from build123d import *

# Parameters (mm, degrees)
F1_DEPTH = 85
F3_D     = 4.2
F3_DEPTH = 14.4
F3_TIP   = 1.2618073
F5_D     = 3.2


with BuildPart() as f1:
    # F0 (on Front) → F1 (new body)
    with BuildSketch(Plane.XZ):
        Polygon((0, 37), (0, 0), (13.5, 0), (13.5, 23), (71.5, 23), (71.5, 0), (85, 0), (85, 37), align=None)
    extrude(amount=F1_DEPTH)

    # F3
    with Locations(Plane.XY.offset(37)):
        with Locations((11.7691496318, -12.5), (72.5, -12.5), (72.5, -72.5), (12.5, -72.5)):
            Hole(F3_D / 2, depth=F3_DEPTH)
            with Locations((0, 0, -(F3_DEPTH + F3_TIP / 2))):  # 118° drill point
                Cone(0, F3_D / 2, F3_TIP, mode=Mode.SUBTRACT)

    # F5 (through all)
    with Locations(Plane.YZ.offset(85)):
        with Locations((-57.5, 19), (-27.5, 19)):
            Hole(F5_D / 2)


solid = f1.part
Design review of the part built by this model. Coordinates are the model's own, in mm. A direction names the side the tool comes from. Give positions to 0.01 mm unless a question says otherwise; leave off trailing zeros. Loops run counter-clockwise (first coordinate to the right, second up) from the corner with the lowest first, then second, coordinate; pieces in that order, holes last. Notation, with made-up numbers: (63, 70.5) - (83, 70.5) arc R14 cw to (83, 83.5) - close; hole circle Ø1 at (-28.5, 54.5). An arc over 180 degrees is marked (long way). Use CSV: the item, a comma, the result in double quotes. Start each with the question number.
1. Add section A-A (y = -57.5). State the section outline as (x, z) points.
2. Wall thickness on L1, parallel to X at y = -12.5, z = 31.75; L2, parallel to X at y = -38.5, z = 18; L3, parallel to Z at x = 37, y = -67: over which ranges is each line inside the solid? List them lowest first.
3. Add section D-D (y = -36). State the section outline as (x, z) points, plus the area to 3 significant figures.
4. Insertion check: P1, Ø2.5, axis at x = 11.77, y = -12.5, coming from the +Z side; P2, Ø1.5, axis at x = 23.5, y = -71.5, coming from the -Z side. Each pin has a flat end and moves straight along its axis. Give the tip position at first contact, or say it passes through.
5. Add section C-C (z = 3.5). State the section outline as (x, y) points.
6. Draft analysis for pull direction Y (two halves, no side actions). For faces 4 (the cylindrical face through (9.766, -11.869, 29.699)), 5 (the flat face through (42, 0, 27)), 6 (the flat face through (42, -42, 23)), state which applies: released by +Y, released by -Y, zero draft, split by the parting line, or undercut.
7. Machinability: for faces 1 (the flat face through (85, -42, 18)), 2 (the flat face through (13.5, -42, 11)), 3 (the cylindrical face through (74.6, -12.41, 29.7)), which of the approach directions +Z, -Z, +X, -X, +Y, -Y give a long, thin tool a straight path to every point of the face, cutting with its end or side? Answer none if there is none.
8. Add section B-B (z = 19). State the section outline as (x, y) points, plus the area to 3 significant figures.
Results found:
1,outline,"(0, 0) - (13.5, 0) - (13.5, 17.4) - (0, 17.4) - close; (0, 20.6) - (13.5, 20.6) - (13.5, 23) - (71.5, 23) - (71.5, 20.6) - (85, 20.6) - (85, 37) - (0, 37) - close; (71.5, 0) - (85, 0) - (85, 17.4) - (71.5, 17.4) - close"
2,L1,"x = 0 to 9.67, 13.87 to 70.4, 74.6 to 85"
2,L2,"x = 0 to 13.5, 71.5 to 85"
2,L3,"z = 23 to 37"
3,outline,"(0, 0) - (13.5, 0) - (13.5, 23) - (71.5, 23) - (71.5, 0) - (85, 0) - (85, 37) - (0, 37) - close"
3,area,"1,810 mm²"
4,P1,"stops at z = 22.09"
4,P2,"stops at z = 23"
5,outline,"(0, -85) - (13.5, -85) - (13.5, 0) - (0, 0) - close; (71.5, -85) - (85, -85) - (85, 0) - (71.5, 0) - close"
6,face 4,"undercut"
6,face 5,"released by +Y"
6,face 6,"zero draft"
7,face 1,"+Z, -Z, +X, +Y, -Y"
7,face 2,"-Z, +Y, -Y"
7,face 3,"+Z"
8,outline,"(0, -85) - (13.5, -85) - (13.5, -59.1) - (0, -59.1) - close; (0, -55.9) - (13.5, -55.9) - (13.5, -29.1) - (0, -29.1) - close; (0, -25.9) - (13.5, -25.9) - (13.5, 0) - (0, 0) - close; (71.5, -85) - (85, -85) - (85, -59.1) - (71.5, -59.1) - close; (71.5, -55.9) - (85, -55.9) - (85, -29.1) - (71.5, -29.1) - close; (71.5, -25.9) - (85, -25.9) - (85, 0) - (71.5, 0) - close"
8,area,"2,120 mm²"
